The model under review builds one solid part; all positions refer to its coordinate system, in mm. Face numbers are marked on the shaded views. A direction names the side the tool comes from. Round coordinates to 2 decimals unless told otherwise and drop trailing zeros. Loops run counter-clockwise (first coordinate to the right, second up) from the corner with the lowest first, then second, coordinate; pieces in that order, holes last. Notation, with made-up numbers: M 10.25,17 L 39.25,17 A17 cw 39.25,46 Z; hole C 50.5,86.25 d6. An arc over 180 degrees is marked long. Answer as a JSON object with one key per item and string values. Group by question number.
Item 1: Consider section B-B (y = -5.25). Give the boundary of the cut face in (x, z) (1 decimal).
Item 2: Tool access review of the marked faces 1, 2 and 3: name each direction out of +Z, -Z, +X, -X, +Y, -Y from which nothing blocks a thin tool from reaching the whole face with its end or side.
Item 3: Consider section A-A (x = 0). Give the boundary of the cut face in (y, z) (1 decimal), and give its area (3 significant figures).
Item 4: Consider section D-D (x = 10). Give the boundary of the cut face in (y, z), and give its area (3 significant figures).
Item 5: Consider section C-C (z = 7). Give the boundary of the cut face in (x, y) (1 decimal).
Item 6: Insertion check: P1, Ø1, axis at x = -2, z = 3, coming from the -Y side; P2, Ø13, axis at x = 0, y = 0, coming from the +Z side; P3, Ø6.5, axis at x = -0.5, y = 3, coming from the -Z side (3 decimals); P4, Ø6, axis at y = 3, z = 3, coming from the -X side. Each pin has a flat end and moves straight along its axis. Give the tip position at first contact, or say it passes through.
Item 7: The part is to be moulded in two halves that separate along Y. For the marked faces 4, 5 and 6, say which applies: +Y half, -Y half, draft (parallel to the pull), parting line (faces both ways), or undercut.
Item 8: To check wall thickness, follow line 1 (Z direction, x = -4.25, y = -9); line 2 (Y direction, x = 0, z = 5.5); line 3 (Y direction, x = 0, z = 1.55) (3 decimals). State the ranges of each line that lie inside material, in increasing order.
```python
from build123d import *

# Parameters (mm, degrees)
F0_R     = 11.1749967
F0_R_2   = 8
F1_DEPTH = 1.5875
F2_R     = 9.5874967
F2_R_2   = 8
F3_DEPTH = 3.41249
F4_R     = 9.5874967
F4_R_2   = 6.4124967
F5_DEPTH = 1.5875
F6_R     = 9.5874967
F6_R_2   = 8
F7_DEPTH = 2.0000214
F8_R     = 11.1749967
F8_R_2   = 8
F9_DEPTH = 2.9999686


with BuildPart() as f1:
    # F0 (on Top) → F1 (new body)
    with BuildSketch(Plane.XY):
        Circle(F0_R)
        Circle(F0_R_2, mode=Mode.SUBTRACT)
    extrude(amount=F1_DEPTH)

    # F2 (on face) → F3 (join)
    with BuildSketch(Plane.XY.offset(1.5875)):
        Circle(F2_R)
        Circle(F2_R_2, mode=Mode.SUBTRACT)
    extrude(amount=F3_DEPTH)

    # F4 (on face) → F5 (join)
    with BuildSketch(Plane.XY.offset(4.99999)):
        Circle(F4_R)
        Circle(F4_R_2, mode=Mode.SUBTRACT)
    extrude(amount=F5_DEPTH)

    # F6 (on face) → F7 (join)
    with BuildSketch(Plane.XY.offset(6.58749)):
        Circle(F6_R)
        Circle(F6_R_2, mode=Mode.SUBTRACT)
    extrude(amount=F7_DEPTH)

    # F8 (on face) → F9 (join)
    with BuildSketch(Plane.XY.offset(8.5875114)):
        Circle(F8_R)
        Circle(F8_R_2, mode=Mode.SUBTRACT)
    extrude(amount=F9_DEPTH)


solid = f1.part
```
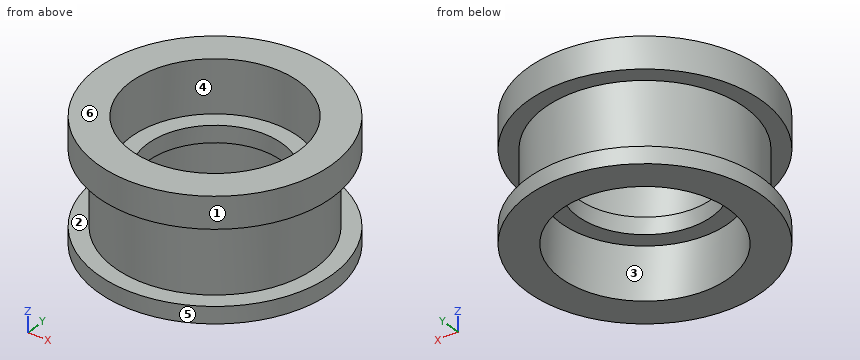
Geometry results:
{
 "1": {"outline": "M -9.9,0 L -6,0 L -6,5 L -3.7,5 L -3.7,6.6 L -6,6.6 L -6,11.6 L -9.9,11.6 L -9.9,8.6 L -8,8.6 L -8,1.6 L -9.9,1.6 Z; M 3.7,5 L 6,5 L 6,0 L 9.9,0 L 9.9,1.6 L 8,1.6 L 8,8.6 L 9.9,8.6 L 9.9,11.6 L 6,11.6 L 6,6.6 L 3.7,6.6 Z"},
 "2": {"face 1": "+Z, -Z", "face 2": "none", "face 3": "-Z"},
 "3": {"outline": "M -11.2,0 L -8,0 L -8,5 L -6.4,5 L -6.4,6.6 L -8,6.6 L -8,11.6 L -11.2,11.6 L -11.2,8.6 L -9.6,8.6 L -9.6,1.6 L -11.2,1.6 Z; M 6.4,5 L 8,5 L 8,0 L 11.2,0 L 11.2,1.6 L 9.6,1.6 L 9.6,8.6 L 11.2,8.6 L 11.2,11.6 L 8,11.6 L 8,6.6 L 6.4,6.6 Z", "area": "56.4 mm^2"},
 "4": {"outline": "M -4.99,0 L 4.99,0 L 4.99,1.59 L -4.99,1.59 Z; M -4.99,8.59 L 4.99,8.59 L 4.99,11.59 L -4.99,11.59 Z", "area": "45.8 mm^2"},
 "5": {"outline": "C 0,0 d19.2; hole C 0,0 d16"},
 "6": {"P1": "stops at y = -9.47", "P2": "stops at z = 6.59", "P3": "passes through", "P4": "stops at x = -11.17"},
 "7": {"face 4": "undercut", "face 5": "parting line", "face 6": "draft"},
 "8": {"line 1": "z = 0 to 1.59, 8.59 to 11.59", "line 2": "y = -9.59 to -6.41, 6.41 to 9.59", "line 3": "y = -11.175 to -8, 8 to 11.175"}
}
